The model under review builds one solid part; all positions refer to its coordinate system, in mm. A direction names the side the tool comes from. Round coordinates to 2 decimals unless told otherwise and drop trailing zeros. Write each loop counter-clockwise with the first axis right and the second up, starting at its lowest first coordinate (ties: lowest second). Pieces come first, ordered by that corner, then holes. Notation, with made-up numbers: (-11, -34.5) -> (7, -34.5) arc R22 cw to (7, -3.5) -> close; hole circle Ø2 at (-17, -32). An arc over 180 degrees is marked (long way). Answer in a Markdown table with one row per item. Add a question column.
Autodesk Inventor part; units mm, degrees
ref_plane "YZ Plane" through (0, 0, 0) normal (1, 0, 0) x (0, 1, 0)
ref_plane "XZ Plane" through (0, 0, 0) normal (0, 1, 0) x (-1, 0, 0)
ref_plane "XY Plane" through (0, 0, 0) normal (0, 0, 1) x (1, 0, 0)
sketch "Esquisse1" plane through (0, 0, 0) normal (0, 1, 0) x (-1, 0, 0)
  arc A0 (58, 0) -> (-58, 0) centre (0, 0) ccw
  arc A1 (68, 0) -> (-68, 0) centre (0, 0) ccw
  line L0 (58, 0) -> (68, 0)
  circle A2 centre (-78, 0) radius 10
  circle A3 centre (-78, 0) radius 1.5
  line L1 (-78, 10) -> (-58.201, 10) construction
  line L2 (-78, 10) -> (-63.6239, 24)
  line L3 (-78, -10) -> (-58, -10)
  line L4 (-58, 0) -> (-58, -10)
  dimension "d9" = 58
  dimension "d10" = 68
  dimension "d11" = 20
  dimension "d12" = 20
  dimension "d13" = 3
extrude "Extrusion1" add sketch "Esquisse1" along normal blind 7
sketch "Esquisse2" plane through (0, 0, 0) normal (0, -1, 0) x (1, 0, 0)
  circle A0 centre (78, 0) radius 2.6
  point P0 (0, 0)
  dimension "d16" = 5.2
extrude "Extrusion2" cut sketch "Esquisse2" against normal blind 4
fillet "Congé1" radius 12 1 edges at (58, 3.5, -10)
fillet "Congé2" radius 2 2 edges at (-68, 3.5, 0) (-58, 3.5, 0)
properties part number "bras_pince_gauche"
1. Add section A-A on z = 18. Write out the cut boundary in (x, y).
2. Add section B-B on x = 0. Write out the cut boundary in (y, z), plus the area to 3 significant figures.
3. For L1, parallel to Z at x = 78, y = 2.7; L2, parallel to Z at x = 78, y = 6.3; L3, parallel to X at y = 2.25, z = 42, list the stretches that pass through material, from the lowest coordinate up.
4. Add section C-C on z = 52. Write out the cut boundary in (x, y), plus the area to 3 significant figures.
5. Insertion check: pin 1 Ø7 at (x, z) = (78, 0) entering from -Y; pin 2 Ø4 at (y, z) = (2.5, 27) entering from -X; pin 3 Ø1.5 at (x, y) = (-19, 1.5) entering from +Z; pin 4 Ø3 at (x, y) = (-62.5, 2) entering from -Z. Each pin has a flat end and moves straight along its axis. Give the tip position at first contact, or say it passes through.
6. Mouldability with a two-part tool opening along X and no side actions: class faces 4 (the cylindrical face through (88, 3, 0)), 5 (the cylindrical face through (1.388, 3.451, 57.983)), 6 (the flat face through (28, 0, 52)) as pulls with the +X half, pulls with the -X half, needs draft (parallel to the pull), parting line crosses it, or undercut.
7. Add section D-D on x = 53. Write out the cut boundary in (y, z), plus the area to 3 significant figures.
8. Tool access review of faces 1 (the flat face through (-63, 3, 0)), 2 (the flat face through (74, 3, -10)), 3 (the flat face through (80, 4, 0)): name each direction out of +Z, -Z, +X, -X, +Y, -Y from which nothing blocks a thin tool from reaching the whole face with its end or side.
Filled in:
| question | item | result |
|---|---|---|
| 1 | outline | (-65.57, 0) -> (-55.14, 0) -> (-55.14, 7) -> (-65.57, 7) -> close; (55.14, 0) -> (69.79, 0) -> (69.79, 7) -> (55.14, 7) -> close |
| 2 | outline | (0, 58) -> (7, 58) -> (7, 68) -> (0, 68) -> close |
| 2 | area | 70.0 mm² |
| 3 | L1 | -10 to -2.6, 2.6 to 10 |
| 3 | L2 | -10 to -1.5, 1.5 to 10 |
| 3 | L3 | -53.48 to -40, 40 to 53.48 |
| 4 | outline | (-43.82, 0) -> (-25.69, 0) -> (-25.69, 7) -> (-43.82, 7) -> close; (25.69, 0) -> (43.82, 0) -> (43.82, 7) -> (25.69, 7) -> close |
| 4 | area | 254 mm² |
| 5 | pin 1 | y = 0 |
| 5 | pin 2 | x = -63.24 |
| 5 | pin 3 | z = 65.51 |
| 5 | pin 4 | z = 0 |
| 6 | face 4 | pulls with the +X half |
| 6 | face 5 | undercut |
| 6 | face 6 | needs draft |
| 7 | outline | (0, 23.56) -> (7, 23.56) -> (7, 42.6) -> (0, 42.6) -> close |
| 7 | area | 133 mm² |
| 8 | face 1 | -Z, -X, +Y, -Y |
| 8 | face 2 | -Z, +X, -X, +Y, -Y |
| 8 | face 3 | -Y |
